Geometry check sheet. Reference: the model listing, model coordinates, mm. A direction names the side the tool comes from. Give positions to 0.01 mm unless a question says otherwise; leave off trailing zeros. Write each loop counter-clockwise with the first axis right and the second up, starting at its lowest first coordinate (ties: lowest second). Pieces come first, ordered by that corner, then holes. Notation, with made-up numbers: M 32.25,-16.5 L 41.25,-16.5 A25 ccw 41.25,0.5 Z; hole C 29.5,85.5 d10. An arc over 180 degrees is marked long. One line per item, written item: value. Start each with the question number.
1. Gauge pin test, flat ends, axial feed: pin 1 (19.5 mm diameter, centred on x = -13, y = 35, fed in from +Z); pin 2 (2.5 mm diameter, centred on x = 0, y = 50, fed in from +Z). Record the tip position at first contact, or that the pin passes through.
2. Cross-section at A-A on y = 50. Record the cut outline in (x, z), then the cut area to 3 significant figures.
3. Cross-section at B-B on z = 2.85. Count the separate pieces of the cut face and the enclosed holes in it, then the cut area to 3 significant figures.
4. Tool access check on faces 1 (the face through (27.49, 25.276, 2.986)), 2 (the face through (71.026, 50.481, 1.972)). Record the directions out of +Z, -Z, +X, -X, +Y, -Y that give a thin tool (end or side, any length) a straight path to the whole face; none if there is none.
5. Cross-section at D-D on x = 43. Record the cut outline in (y, z).
6. Scan lines: line 1 (Y direction, x = 69.5, z = 0.8); line 2 (Y direction, x = 0, z = 2.5); line 3 (X direction, y = 0, z = 2.4). Record each from-to range of solid material in increasing order.
7. Cross-section at C-C on x = -69.5. Record the cut outline in (y, z).
8. Release check for a two-part mould opening along Y. For faces 3 (the face through (-67.974, -49.519, 1.972)), 4 (the face through (-1, 55, 2)), 5 (the face through (74.5, -1, 2)), 6 (the face through (27.49, -25.276, 2.986)) record: pulls with the +Y half, pulls with the -Y half, needs draft (parallel to the pull), parting line crosses it, or undercut.
from build123d import *

# Parameters (mm, degrees)
SKICA1_W                = 149
SKICA1_H                = 110
SKICA1_R                = 1.6
P_IDAT_VYSUNUT_M1_DEPTH = 2
SKICA2_W                = 149
SKICA2_H                = 110
SKICA2_R                = 1.6
P_IDAT_VYSUNUT_M2_DEPTH = 2
ZAOBLIT1_R              = 2


with BuildPart() as part:
    # Skica1 → Přidat vysunutím1 (new body)
    with BuildSketch(Plane.XY):
        Rectangle(SKICA1_W, SKICA1_H)
        with Locations((-69.5, 50)):
            Circle(SKICA1_R, mode=Mode.SUBTRACT)
        with Locations((69.5, 50)):
            Circle(SKICA1_R, mode=Mode.SUBTRACT)
        with Locations((69.5, -50)):
            Circle(SKICA1_R, mode=Mode.SUBTRACT)
        with Locations((-69.5, -50)):
            Circle(SKICA1_R, mode=Mode.SUBTRACT)
        with Locations((0, 50)):
            Circle(SKICA1_R, mode=Mode.SUBTRACT)
        with Locations((0, -50)):
            Circle(SKICA1_R, mode=Mode.SUBTRACT)
    extrude(amount=P_IDAT_VYSUNUT_M1_DEPTH)

    # Skica2 → Přidat vysunutím2 (add)
    with BuildSketch(Plane.XY.offset(2)):
        Rectangle(SKICA2_W, SKICA2_H)
        with Locations((-69.5, -50)):
            Circle(SKICA2_R, mode=Mode.SUBTRACT)
        with Locations((69.5, -50)):
            Circle(SKICA2_R, mode=Mode.SUBTRACT)
        with Locations((69.5, 50)):
            Circle(SKICA2_R, mode=Mode.SUBTRACT)
        with Locations((-69.5, 50)):
            Circle(SKICA2_R, mode=Mode.SUBTRACT)
        with Locations((0, -50)):
            Circle(SKICA2_R, mode=Mode.SUBTRACT)
        with Locations((0, 50)):
            Circle(SKICA2_R, mode=Mode.SUBTRACT)
        Polygon((55.761515514, -45), (-55.761515514, -45), (0, -6.096617083), align=None, mode=Mode.SUBTRACT)
        Polygon((64.5, -38.903382917), (64.5, 38.903382917), (8.738484486, 0), align=None, mode=Mode.SUBTRACT)
        Polygon((55.761515514, 45), (-55.761515514, 45), (0, 6.096617083), align=None, mode=Mode.SUBTRACT)
        Polygon((-64.5, -38.903382917), (-64.5, 38.903382917), (-8.738484486, 0), align=None, mode=Mode.SUBTRACT)
    extrude(amount=P_IDAT_VYSUNUT_M2_DEPTH)

    # Zaoblit1
    zaoblit1_edges = [part.edges().sort_by_distance(p)[0] for p in [
        (74.5, -55, 2),
        (-74.5, -55, 2),
        (-74.5, 55, 2),
        (74.5, 55, 2),
    ]]
    fillet(zaoblit1_edges, radius=ZAOBLIT1_R)


solid = part.part
Report:
1. pin 1: stops at z = 2
1. pin 2: passes through
2. outline: M -74.5,0 L -71.1,0 L -71.1,4 L -74.5,4 Z; M -67.9,0 L -1.6,0 L -1.6,4 L -67.9,4 Z; M 1.6,0 L 67.9,0 L 67.9,4 L 1.6,4 Z; M 71.1,0 L 74.5,0 L 74.5,4 L 71.1,4 Z
2. area: 558 mm^2
3. separate pieces: 1
3. enclosed holes: 10
3. area: 7,660 mm^2
4. face 1: +Z
4. face 2: +Z, -Z
5. outline: M -55,0 L 55,0 L 55,4 L 45,4 L 45,2 L 36.1,2 L 36.1,4 L 23.9,4 L 23.9,2 L -23.9,2 L -23.9,4 L -36.1,4 L -36.1,2 L -45,2 L -45,4 L -55,4 Z
6. line 1: y = -55 to -51.6, -48.4 to 48.4, 51.6 to 55
6. line 2: y = -55 to -51.6, -48.4 to -45, -6.1 to 6.1, 45 to 48.4, 51.6 to 55
6. line 3: x = -74.5 to -64.5, -8.74 to 8.74, 64.5 to 74.5
7. outline: M -55,0 L -51.6,0 L -51.6,4 L -55,4 Z; M -48.4,0 L 48.4,0 L 48.4,4 L -48.4,4 Z; M 51.6,0 L 55,0 L 55,4 L 51.6,4 Z
8. face 3: undercut
8. face 4: pulls with the +Y half
8. face 5: needs draft
8. face 6: undercut
